```python
from build123d import *

# Parameters (mm, degrees)
SKETCH1_W           = 20
SKETCH1_H           = 20
BOSS_EXTRUDE1_DEPTH = 9.5
CUT_EXTRUDE1_REACH  = 22
SKETCH3_R           = 2.6
CHAMFER1_SIZE       = 1


with BuildPart() as part:
    # Sketch1 → Boss-Extrude1 (new body)
    with BuildSketch(Plane(origin=(0, 0, 0), x_dir=(1, 0, 0), z_dir=(0, 1, 0))):
        Rectangle(SKETCH1_W, SKETCH1_H)
        with BuildLine():
            Line((-5.319354919, 3.821905708), (-3, 7.05))
            Line((-3, 7.05), (3, 7.05))
            Line((3, 7.05), (5.319354919, 3.821905708))
            ThreePointArc((5.319354919, 3.821905708), (0, -6.55), (-5.319354919, 3.821905708))
        make_face(mode=Mode.SUBTRACT)
    extrude(amount=BOSS_EXTRUDE1_DEPTH)

    # Sketch3 → Cut-Extrude1 (cut, up to next)
    with BuildSketch(Plane(origin=(0, 0, -10), x_dir=(-1, 0, 0), z_dir=(0, 0, -1)), mode=Mode.PRIVATE) as cut_extrude1_sk1:
        with Locations((0, 4.75)):
            Circle(SKETCH3_R)
    cut_extrude1_tool1 = extrude(cut_extrude1_sk1.sketch, amount=-CUT_EXTRUDE1_REACH, mode=Mode.PRIVATE) & part.part
    add(cut_extrude1_tool1.solids().sort_by_distance((0, 4.75, -10))[0], mode=Mode.SUBTRACT)

    # Chamfer1
    chamfer1_edges = [part.edges().sort_by_distance(p)[0] for p in [
        (-10, 4.75, -10),
        (10, 4.75, -10),
        (10, 4.75, 10),
        (-10, 4.75, 10),
    ]]
    chamfer(chamfer1_edges, length=CHAMFER1_SIZE)


solid = part.part
```
Input: part model. Units: mm. Frame: model coordinates. A direction names the side the tool comes from. Round coordinates to 2 decimals unless told otherwise and drop trailing zeros. Loops run counter-clockwise (first coordinate to the right, second up) from the corner with the lowest first, then second, coordinate; pieces in that order, holes last. Notation, with made-up numbers: (16.25, -5) -> (67.25, -5) arc R24 cw to (67.25, 15) -> close; hole circle Ø1 at (56, -31). An arc over 180 degrees is marked (long way). One line per item, written item: value.
(1) Section B-B (z = 0). Return the cut outline in (x, y), plus the area to 4 significant figures.
Geometry check:
outline: (-10, 0) -> (-6.55, 0) -> (-6.55, 9.5) -> (-10, 9.5) -> close; (6.55, 0) -> (10, 0) -> (10, 9.5) -> (6.55, 9.5) -> close
area: 65.55 mm2
(2) Section D-D (x = -3.5). Return the cut outline in (y, z).
Geometry check:
outline: (0, -10) -> (9.5, -10) -> (9.5, -6.35) -> (0, -6.35) -> close; (0, 5.54) -> (9.5, 5.54) -> (9.5, 10) -> (0, 10) -> close
(3) Section A-A (x = 0). Return the cut outline in (y, z), plus the area to 3 significant figures.
Geometry check:
outline: (0, -10) -> (2.15, -10) -> (2.15, -7.05) -> (0, -7.05) -> close; (0, 6.55) -> (9.5, 6.55) -> (9.5, 10) -> (0, 10) -> close; (7.35, -10) -> (9.5, -10) -> (9.5, -7.05) -> (7.35, -7.05) -> close
area: 45.5 mm2
(4) Pin query (flat end, axial travel): pin 1 (3 mm diameter, centred on x = 3, z = 4.5, fed in from +Y); pin 2 (3 mm diameter, centred on x = 0, y = 4.75, fed in from -Z). Return the tip coordinate at first contact, or that it passes through.
Geometry check:
pin 1: y = 9.5
pin 2: z = 6.38
(5) Material intervals for line 1 (Y direction, x = 0, z = -9.4); line 2 (X direction, y = 6.5, z = 0); line 3 (Z direction, x = -4.75, y = 5.25), sorted ascending. Write a range as [from, to].
Geometry check:
line 1: [0, 2.15], [7.35, 9.5]
line 2: [-10, -6.55], [6.55, 10]
line 3: [-10, -4.61], [4.51, 10]
(6) Set-up query: faces 5 (the face through (0.338, 7.328, -8.546)), 6 (the face through (9.5, 4.7, -9.5)), 7 (the face through (-4.18, 4.68, -5.41)). Return all of +Z, -Z, +X, -X, +Y, -Y with unobstructed straight access to the full face (end or side cutting, diameter ignored); none if empty.
Geometry check:
face 5: -Z
face 6: -Z, +X, +Y, -Y
face 7: +Y, -Y
(7) Mould query, pull axis X, two halves, no side actions, for faces 1 (the face through (9.5, 4.7, 9.5)), 2 (the face through (-9.5, 4.7, 9.5)), 3 (the face through (2.6, 5.7, -7.05)), 4 (the face through (-7, 9.5, 0)). Classes: pulls with the +X half, pulls with the -X half, needs draft (parallel to the pull), parting line crosses it, or undercut.
Geometry check:
face 1: pulls with the +X half
face 2: pulls with the -X half
face 3: undercut
face 4: needs draft
(8) Section C-C (y = 8.75). Return the cut outline in (x, z), plus the area to 3 significant figures.
Geometry check:
outline: (-10, -9) -> (-9, -10) -> (9, -10) -> (10, -9) -> (10, 9) -> (9, 10) -> (-9, 10) -> (-10, 9) -> close; hole (-5.32, -3.82) -> (-3, -7.05) -> (3, -7.05) -> (5.32, -3.82) arc R6.55 ccw (long way) to start
area: 257 mm2
